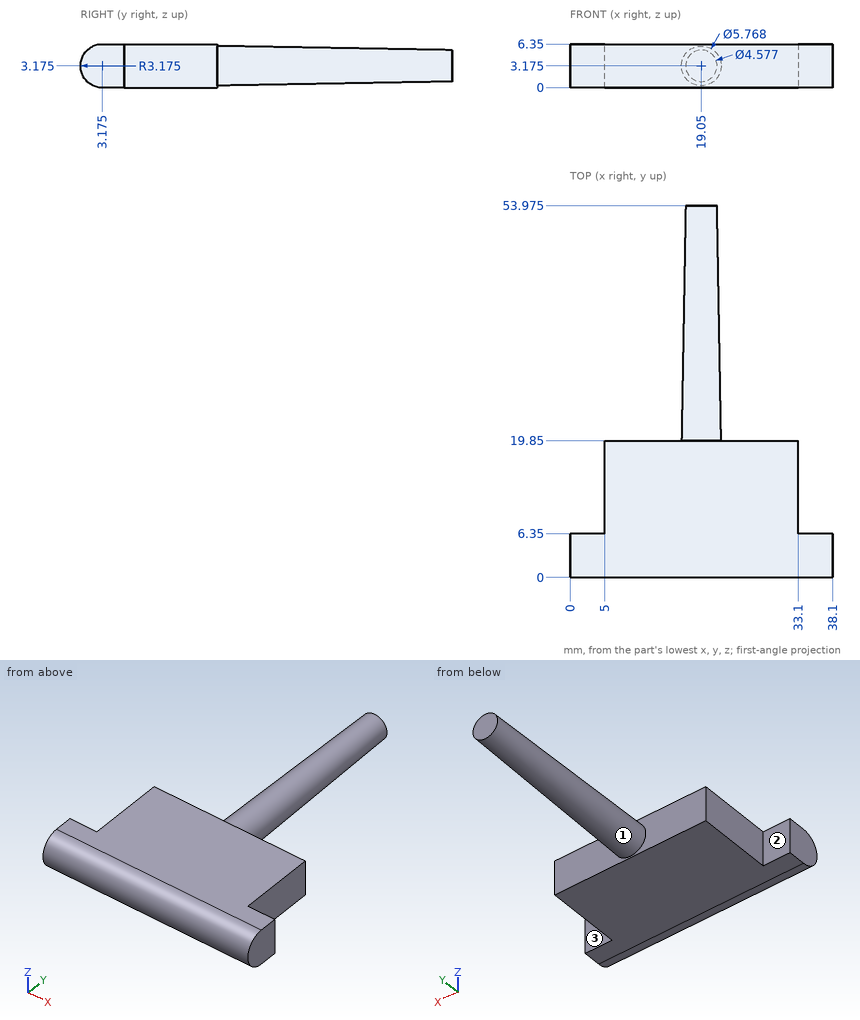
The figure shows three views and two pictorial views of one solid part (mm, origin at its lowest corner). Answer the questions. A direction names the side the tool comes from. Round coordinates to 2 decimals unless told otherwise and drop trailing zeros. Put each result on its own line as item: value.
Q1. Consider line 1 along X through (y, z) = (19, 4.25); line 2 along X through (y, z) = (25.5, 5.5) (1 decimal); line 3 along Y through (x, z) = (13.5, 2.5). Determine where each line is inside the solid, lowest interval first.
Results list:
line 1: 5 to 33.1
line 2: 17.5 to 20.6
line 3: 0.07 to 19.85
Q2. Each of these flat-tipped pins is pushed along its axis until it touches: P1, Ø1, axis at x = 30, z = 5, coming from the -Y side; P2, Ø2, axis at y = 8, z = 1, coming from the +X side; P3, Ø1.5, axis at x = 34.5, z = 2, coming from the +Y side. Where does it stop, or does it pass through?
Results list:
P1: y = 0.29
P2: x = 33.1
P3: y = 6.35
Q3. Which of the six approach directions +Z, -Z, +X, -X, +Y, -Y give full straight-line access (tool end or side, diameter ignored) to the marked faces 1, 2 and 3?
Results list:
face 1: +Y
face 2: +Z, -Z, -X, +Y
face 3: +Z, -Z, +X, +Y
